Could you check a few things on this model? Use its own coordinates, in mm. Face numbers are marked on the shaded views. Give positions to 0.01 mm unless a question says otherwise; leave off trailing zeros. Order: outer loops, then holes, each group sorted by start corner. A loop starts at its lowest first (then second) coordinate and runs counter-clockwise, first axis right, second up. Notation, with made-up numbers: M 32.25,-25 L 47.25,-25 A30 cw 47.25,11 Z; hole C 21.25,-13.5 d8. An arc over 180 degrees is marked long. Use a Markdown table: item, result. Add a question column.
Item 1: If I drill on L1, parallel to Z at x = -6.5, y = 1.9; L2, parallel to X at y = 3.65, z = 13, over which ranges is the centre line in solid material (lowest first)? Write a range as from..to.
Item 2: Suppose I cut it at A-A on y = 1.65. Write out the boundary of the cut face in (x, z).
Item 3: If we mould it in two halves opening along X, with no side actions, what happens to the marked faces 1, 2 and 3? For each: released by +X, released by -X, zero draft, split by the parting line, or undercut.
Item 4: I'm going to push flat-ended pins straight in: pin 1 Ø18.5 at (x, z) = (6, 5) entering from +Y; pin 2 Ø5 at (x, z) = (2, -11.5) entering from -Y; pin 3 Ø2 at (y, z) = (3.5, -12.5) entering from -X. Where does each tip first touch, or does it pass through?
Autodesk Inventor part; units mm, degrees
ref_plane "작업 평면3" through (0, 2.2, 0) normal (0, -1, 0) x (1, 0, 0)
ref_plane "YZ Plane" through (0, 0, 0) normal (1, 0, 0) x (0, 1, 0)
ref_plane "XZ Plane" through (0, 0, 0) normal (0, 1, 0) x (-1, 0, 0)
sketch "스케치1" plane through (0, 0, 0) normal (0, 1, 0) x (-1, 0, 0)
  line L0 (-16.2959, 6.75) -> (-6.75, 16.2959)
  line L1 (-6.75, 16.2959) -> (6.75, 16.2959)
  line L2 (6.75, 16.2959) -> (16.2959, 6.75)
  line L3 (16.2959, 6.75) -> (16.2959, -6.75)
  line L4 (16.2959, -6.75) -> (6.75, -16.2959)
  line L5 (6.75, -16.2959) -> (-6.75, -16.2959)
  line L6 (-6.75, -16.2959) -> (-16.2959, -6.75)
  line L7 (-16.2959, -6.75) -> (-16.2959, 6.75)
  line L8 (18.8959, 7.827) -> (18.8959, -7.827)
  line L9 (18.8959, -7.827) -> (7.827, -18.8959)
  line L10 (7.827, -18.8959) -> (-7.827, -18.8959)
  line L11 (-7.827, -18.8959) -> (-18.8959, -7.827)
  line L12 (-18.8959, -7.827) -> (-18.8959, 7.827)
  line L13 (-18.8959, 7.827) -> (-7.827, 18.8959)
  line L14 (-7.827, 18.8959) -> (7.827, 18.8959)
  line L15 (7.827, 18.8959) -> (18.8959, 7.827)
  point P0 (0, 0)
  point P1 (0, 0)
  point P2 (0, 0)
  dimension "d0" = 13.5
  dimension "d1" = 2.6
extrude "돌출1" add sketch "스케치1" along normal blind 4.4 contours L0 L1 L2 L3 L4 L5 L6 L7 | L8 L9 L10 L11 L12 L13 L14 L15
sketch "스케치14" plane through (0, 4.4, 0) normal (0, 1, 0) x (1, 0, 0)
  line L0 (6.75, -16.2959) -> (-6.75, -16.2959)
  line L1 (-6.75, -16.2959) -> (-16.2959, -6.75)
  line L2 (-16.2959, -6.75) -> (-16.2959, 6.75)
  line L3 (-16.2959, 6.75) -> (-6.75, 16.2959)
  line L4 (-6.75, 16.2959) -> (6.75, 16.2959)
  line L5 (6.75, 16.2959) -> (16.2959, 6.75)
  line L6 (16.2959, 6.75) -> (16.2959, -6.75)
  line L7 (16.2959, -6.75) -> (6.75, -16.2959)
  line L8 (-7.5784, 18.2959) -> (7.5784, 18.2959)
  line L9 (7.5784, 18.2959) -> (18.2959, 7.5784)
  line L10 (18.2959, 7.5784) -> (18.2959, -7.5784)
  line L11 (18.2959, -7.5784) -> (7.5784, -18.2959)
  line L12 (7.5784, -18.2959) -> (-7.5784, -18.2959)
  line L13 (-7.5784, -18.2959) -> (-18.2959, -7.5784)
  line L14 (-18.2959, -7.5784) -> (-18.2959, 7.5784)
  line L15 (-18.2959, 7.5784) -> (-7.5784, 18.2959)
  line L16 (18.8959, -7.827) -> (18.8959, 7.827)
  point P0 (0, 0)
  point P1 (0, 0)
  point P2 (0, 0)
  dimension "d138" = 2
  dimension "d139" = 0.6
extrude "돌출16" cut sketch "스케치14" against normal blind 1.2
sketch "스케치15" plane through (0, 4.4, 0) normal (0, 1, 0) x (1, 0, 0)
  line L0 (-16.2959, -6.75) -> (-6.75, -16.2959)
  line L1 (-6.75, -16.2959) -> (6.75, -16.2959)
  line L2 (6.75, -16.2959) -> (16.2959, -6.75)
  line L3 (16.2959, -6.75) -> (16.2959, 6.75)
  line L4 (16.2959, 6.75) -> (6.75, 16.2959)
  line L5 (6.75, 16.2959) -> (-6.75, 16.2959)
  line L6 (-6.75, 16.2959) -> (-16.2959, 6.75)
  line L7 (-16.2959, 6.75) -> (-16.2959, -6.75)
  point P0 (0, 0)
extrude "돌출17" cut sketch "스케치15" against normal blind 0.6
sketch "스케치16" plane through (0, 3.8, 0) normal (0, 1, 0) x (1, 0, 0)
  line L0 (-6.5015, 15.6959) -> (6.5015, 15.6959)
  line L1 (6.5015, 15.6959) -> (15.6959, 6.5015)
  line L2 (15.6959, 6.5015) -> (15.6959, -6.5015)
  line L3 (15.6959, -6.5015) -> (6.5015, -15.6959)
  line L4 (6.5015, -15.6959) -> (-6.5015, -15.6959)
  line L5 (-6.5015, -15.6959) -> (-15.6959, -6.5015)
  line L6 (-15.6959, -6.5015) -> (-15.6959, 6.5015)
  line L7 (-15.6959, 6.5015) -> (-6.5015, 15.6959)
  line L8 (16.2959, 6.75) -> (16.2959, -6.75)
  point P0 (0, 0)
  point P1 (0, 0)
  dimension "d144" = 0.6
extrude "돌출18" cut sketch "스케치16" against normal up to surface (3.8 mm away)
fillet "모깎기2" radius 0.6 16 edges at (0, 4.4, -18.8959) (-13.3614, 4.4, -13.3614) (13.3614, 4.4, -13.3614) (18.8959, 4.4, 0) (13.3614, 4.4, 13.3614) (0, 4.4, 18.8959) (-13.3614, 4.4, 13.3614) (-18.8959, 4.4, 0) (-18.8959, 0, 0) (-13.3614, 0, 13.3614) (0, 0, 18.8959) (13.3614, 0, 13.3614) (-13.3614, 0, -13.3614) (0, 0, -18.8959) (18.8959, 0, 0) (13.3614, 0, -13.3614)
ref_plane "작업 평면3" through (0, 2.2, 0) normal (0, -1, 0) x (1, 0, 0)
mirror "미러6" about plane through (0, 2.2, 0) normal (0, -1, 0) of "돌출17", "돌출16"
properties part number "OV-PAM_ring_2"
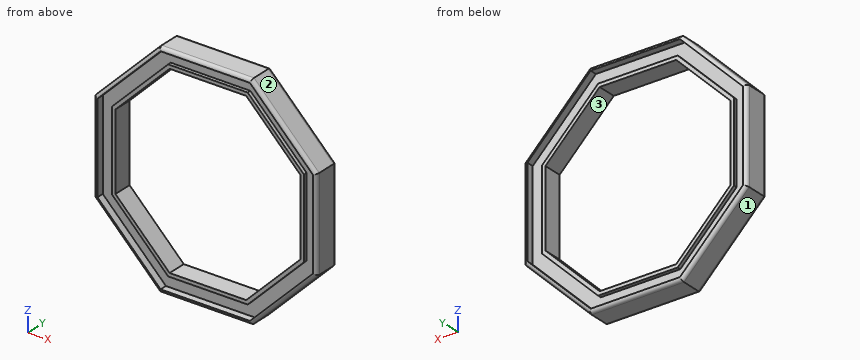
Findings below:
| question | item | result |
|---|---|---|
| 1 | L1 | z = -18.9..-15.7, 15.7..18.9 |
| 1 | L2 | x = -13.72..-12.87, -10.05..-9.2, 9.2..10.05, 12.87..13.72 |
| 2 | outline | M -18.9,-7.83 L -7.83,-18.9 L 7.83,-18.9 L 18.9,-7.83 L 18.9,7.83 L 7.83,18.9 L -7.83,18.9 L -18.9,7.83 Z; hole M -15.7,-6.5 L -6.5,-15.7 L 6.5,-15.7 L 15.7,-6.5 L 15.7,6.5 L 6.5,15.7 L -6.5,15.7 L -15.7,6.5 Z |
| 3 | face 1 | released by -X |
| 3 | face 2 | released by +X |
| 3 | face 3 | undercut |
| 4 | pin 1 | stops at y = 3.8 |
| 4 | pin 2 | passes through |
| 4 | pin 3 | stops at x = -15.22 |
